Read the model definition and answer for the solid it produces. Units are mm, in the model's axes. A direction names the side the tool comes from. Give positions to 0.01 mm unless a question says otherwise; leave off trailing zeros. Order: outer loops, then holes, each group sorted by start corner. A loop starts at its lowest first (then second) coordinate and runs counter-clockwise, first axis right, second up. Notation, with made-up numbers: (57.25, 84.25) -> (114.25, 84.25) arc R11 cw to (114.25, 93.25) -> close; hole circle Ø6 at (-3, -8). An arc over 180 degrees is marked (long way). Use one line per item in the form item = value.
Autodesk Inventor part; units mm, degrees
ref_plane "Work Plane1" through (1.525, 0, 0) normal (0, 0, 1) x (1, 0, 0)
ref_plane "YZ Plane" through (0, 0, 0) normal (1, 0, 0) x (0, 1, 0)
ref_plane "XZ Plane" through (0, 0, 0) normal (0, 1, 0) x (-1, 0, 0)
sketch "Эскиз1" plane through (0, 0, 0) normal (0, 0, 1) x (1, 0, 0)
  line L0 (0, 5) -> (80, 5)
  line L1 (80, 5) -> (80, 0)
  line L2 (80, 0) -> (0, 0)
  line L3 (-16, 0) -> (96, 0)
  line L4 (0, -1) -> (0, 6)
  line L5 (0, 5) -> (0, 0)
  dimension "d2" = 10
  dimension "d59" = 80
revolve "Базовый элемент" add sketch "Эскиз1" angle 360 about axis through (80, 0, 0) along (-1, 0, 0)
sketch "Эскиз2" plane through (0, 0, 0) normal (-1, 0, 0) x (0, 0, 1)
  line L0 (0, 9.2376) -> (8, 4.6188)
  line L1 (8, 4.6188) -> (8, -4.6188)
  line L2 (8, -4.6188) -> (0, -9.2376)
  line L3 (0, -9.2376) -> (-8, -4.6188)
  line L4 (-8, -4.6188) -> (-8, 4.6188)
  line L5 (-8, 4.6188) -> (0, 9.2376)
  line L6 (-11.2, 0) -> (11.2, 0)
  line L7 (0, 12.9326) -> (0, -12.9326)
  point P0 (0, 0)
  point P1 (0, 0)
  dimension "d11" = 16
extrude "С головкой" add sketch "Эскиз2" along normal blind 6.85
sketch "Эскиз4" plane through (0, 0, 0) normal (0, 0, 1) x (1, 0, 0)
  line L0 (-5.9262, 9.6) -> (-6.85, 8)
  line L1 (-1.1, 0) -> (-0.234, 0)
  line L2 (-8.1732, 0) -> (1.0892, 0)
  line L3 (-6.85, 9.6) -> (-5.9262, 9.6)
  line L4 (-6.85, 8) -> (-6.85, 9.6)
  line L5 (0, 11.52) -> (0, -1.92)
  dimension "d65" = 16
  dimension "d67" = 30
  dimension "d68" = 19.2
  dimension "d69" = 6.85
revolve "Фаска1" cut sketch "Эскиз4" angle 360 about axis through (-1.1, 0, 0) along (1, 0, 0)
thread "Резьба"
chamfer "Фаска2" distance 0.9202 distance2 0.9203 1 edges at (80, -5, 0) measured on face at (80, 0.2493, 1.2557)
fillet "Fillet" radius 0.4 1 edges at (0, -5, 0)
ref_plane "Work Plane1" through (1.525, 0, 0) normal (0, 0, 1) x (1, 0, 0)
equation "\"d2\" = GD"
equation "\"d59\" = NLG"
equation "\"d11\" = SW"
equation "\"d3\" = KOH"
equation "\"d71\" = RR1"
equation "\"d15\" = GEL"
equation "\"d6\" = -0.5 * SPD + 0.5 * GD"
equation "\"d65\" = SW"
equation "\"d67\" = ANG1"
equation "\"d68\" = 1.2 * SW"
equation "\"d69\" = KOH"
equation "\"NLG\" = 80"
equation "\"GD\" = NND"
equation "\"KOH\" = 6.85"
equation "\"GEL\" = 26"
equation "\"SW\" = 16"
equation "\"SW0\" = SW"
equation "\"SPD\" = NND - 1.2269 * PTC"
equation "\"SD\" = 0"
equation "\"ANG1\" = 30deg"
equation "\"GAL\" = 0.61345 * PTC"
equation "\"GUL\" = 0.61345 * PTC"
equation "\"RR\" = 0.1"
equation "\"RR1\" = 0.4"
equation "\"GD1\" = THREADDIA - 1.2269 * PTC"
equation "\"TOA\" = 30deg"
equation "\"PTC\" = 1.5"
equation "\"KOH1\" = 4.5"
equation "\"E0\" = 1.155 * SW"
properties part number "ANSI B18.2.3.5M - M10 x 1,5 x 80" material "Сталь, мягкая"
Item 1: Straight lines are drawn through the part: L1, parallel to X at y = -5, z = 5; L2, parallel to Y at x = 14, z = -3. For each, find the intervals that lie inside material, in ascending order. Write a range as from..to.
Checks:
L1 = -6.85..0
L2 = -4..4
Item 2: The part is cut by section A-A on x = 33. Give the vertices of the cut face in (y, z).
Checks:
outline = circle Ø10 at (0, 0)
Item 3: Given pin 1 Ø4 at (x, y) = (51, 2) entering from -Z; pin 2 Ø1.5 at (y, z) = (-3, 4.5) entering from +X; pin 3 Ø3 at (x, y) = (2.5, 6) entering from +Z, each flat-ended and moving along its own axis, determine where each tip first touches the part or whether it passes through.
Checks:
pin_1 = -5
pin_2 = 79.42
pin_3 = 2.18
Item 4: Which of the six approach directions +Z, -Z, +X, -X, +Y, -Y give full straight-line access (tool end or side, diameter ignored) to faces 1 (the cylindrical face through (40.29, -1.08, -4.88)), 2 (the conical face through (-6.676, -4.168, -7.179))?
Checks:
face_1 = +X
face_2 = -Z, -X, -Y
